```python
from build123d import *

# Parameters (mm, degrees)
F0_R     = 1.7272
F0_R_2   = 3.96875
F0_R_3   = 11.1125
F0_R_4   = 2.15265
F1_DEPTH = 3.175
F3_DEPTH = 3.175
F4_COUNT = 6
F4_ANGLE = 300


with BuildPart() as f1:
    # F0 (on Top) → F1 (new body)
    with BuildSketch(Plane.XY):
        with BuildLine():
            Line((-303.6125627, 32.54375), (-346.1094200534, 21.5120031198))
            ThreePointArc((-346.1094200534, 21.5120031198), (-362.7501254, 0), (-346.1094200534, -21.5120031198))
            Line((-346.1094200534, -21.5120031198), (-303.6125627, -32.54375))
            Line((-303.6125627, -32.54375), (-297.2625627, -32.54375))
            Line((-297.2625627, -32.54375), (-297.2625627, -29.36875))
            Line((-297.2625627, -29.36875), (-43.2625627, -29.36875))
            Line((-43.2625627, -29.36875), (-43.2625627, -32.54375))
            Line((-43.2625627, -32.54375), (-36.9125627, -32.54375))
            Line((-36.9125627, -32.54375), (5.5842946534, -21.5120031198))
            ThreePointArc((5.5842946534, -21.5120031198), (22.225, 0), (5.5842946534, 21.5120031198))
            Line((5.5842946534, 21.5120031198), (-36.9125627, 32.54375))
            Line((-36.9125627, 32.54375), (-43.2625627, 32.54375))
            Line((-43.2625627, 32.54375), (-43.2625627, 29.36875))
            Line((-43.2625627, 29.36875), (-297.2625627, 29.36875))
            Line((-297.2625627, 29.36875), (-297.2625627, 32.54375))
            Line((-297.2625627, 32.54375), (-303.6125627, 32.54375))
        make_face()
        with Locations((-282.9750627, -24.60625)):
            Circle(F0_R, mode=Mode.SUBTRACT)
        with Locations((-352.3117115589, -11.7865861589)):
            Circle(F0_R, mode=Mode.SUBTRACT)
        with Locations((-328.7385392411, -11.7865861589)):
            Circle(F0_R_2, mode=Mode.SUBTRACT)
        with Locations((-57.5500627, -24.60625)):
            Circle(F0_R, mode=Mode.SUBTRACT)
        with Locations((-11.7865861589, -11.7865861589)):
            Circle(F0_R_2, mode=Mode.SUBTRACT)
        with Locations((11.7865861589, -11.7865861589)):
            Circle(F0_R, mode=Mode.SUBTRACT)
        with Locations((-340.5251254, 0)):
            Circle(F0_R_3, mode=Mode.SUBTRACT)
        with Locations((-289.7251254, 0)):
            Circle(F0_R_4, mode=Mode.SUBTRACT)
        with Locations((-352.3117115589, 11.7865861589)):
            Circle(F0_R_2, mode=Mode.SUBTRACT)
        with Locations((-328.7385392411, 11.7865861589)):
            Circle(F0_R, mode=Mode.SUBTRACT)
        with Locations((-282.9750627, 24.60625)):
            Circle(F0_R, mode=Mode.SUBTRACT)
        with Locations((-50.8, 0)):
            Circle(F0_R_4, mode=Mode.SUBTRACT)
        Circle(F0_R_3, mode=Mode.SUBTRACT)
        with Locations((-11.7865861589, 11.7865861589)):
            Circle(F0_R, mode=Mode.SUBTRACT)
        with Locations((11.7865861589, 11.7865861589)):
            Circle(F0_R_2, mode=Mode.SUBTRACT)
        with Locations((-57.5500627, 24.60625)):
            Circle(F0_R, mode=Mode.SUBTRACT)
    extrude(amount=F1_DEPTH)

    # F2 (on face) → F3 (cut, through all)
    with BuildSketch(Plane(origin=(0, 0, 0), x_dir=(1, 0, 0), z_dir=(0, 0, -1))):
        with BuildLine():
            ThreePointArc((-348.3828495059, -7.8577241059), (-350.1488326996, -5.55625), (-351.2589761446, -2.8761266387))
            Line((-351.2589761446, -2.8761266387), (-352.0256797693, -3.0815642558))
            ThreePointArc((-352.0256797693, -3.0815642558), (-350.8362403638, -5.953125), (-348.9441155135, -8.4189901135))
            Line((-348.9441155135, -8.4189901135), (-348.3828495059, -7.8577241059))
        make_face()
    f3 = extrude(amount=-F3_DEPTH, mode=Mode.SUBTRACT)

    # F4: F3 ×6 about axis
    f4_axis = Axis((-340.5251254, 0, 0), (0, 0, -1))
    for i in range(1, F4_COUNT):
        add(f3.rotate(f4_axis, i * F4_ANGLE / (F4_COUNT - 1)), mode=Mode.SUBTRACT)


solid = f1.part
```
Here's how the part is built. I have some questions about the finished solid (model axes, mm). Give positions to 0.01 mm unless a question says otherwise; leave off trailing zeros. Order: outer loops, then holes, each group sorted by start corner. A loop starts at its lowest first (then second) coordinate and runs counter-clockwise, first axis right, second up. Notation, with made-up numbers: M 45,-4.5 L 72,-4.5 A28 ccw 72,34.5 Z; hole C 65.5,-12 d10. An arc over 180 degrees is marked long. Use a Markdown table: item, result. Add a question column.
1. I need wall thicknesses on probe 1 along Y at (x, z) = (0.5, 0.8); probe 2 along X at (y, z) = (0.5, 2.95); probe 3 along X at (y, z) = (5, 1.5). Which ranges of each line are inside material? Lowest first, please. Write a range as from..to.
2. Suppose I cut it at A-A (x = 0). List the corners of the cut face in (y, z) for me (1 decimal).
3. Suppose I cut it at B-B (z = 1.7). Give the number of separate pieces and of enclosed holes in the cut face, and give its area (3 significant figures).
4. Suppose I cut it at C-C (x = -207.5). List the corners of the cut face in (y, z) for me (3 decimals), and give its area (3 significant figures).
5. If we mould it in two halves opening along Z, with no side actions, what happens to faces 1 (the cylindrical face through (10.6, 3.34, 1.57)), 2 (the flat face through (-173, 0, 3.175)), 3 (the flat face through (-173, 0, 0))? For each: +Z half, -Z half, draft (parallel to the pull), parting line (faces both ways), or undercut.
6. For pin 1 Ø5.5 at (x, y) = (-282.98, 24.61) entering from -Z; pin 2 Ø18 at (x, y) = (0, 0) entering from -Z, each with a flat end and sliding along its axis, tell me the tip position at first contact or that it passes through.
Results list:
| question | item | result |
|---|---|---|
| 1 | probe 1 | y = -22.83..-11.1, 11.1..22.83 |
| 1 | probe 2 | x = -362.74..-351.63, -329.42..-291.82, -287.63..-52.89, -48.71..-11.1, 11.1..22.22 |
| 1 | probe 3 | x = -362.18..-351.33, -329.72..-9.92, 9.92..21.66 |
| 2 | outline | M -23,0 L -11.1,0 L -11.1,3.2 L -23,3.2 Z; M 11.1,0 L 23,0 L 23,3.2 L 11.1,3.2 Z |
| 3 | separate pieces | 1 |
| 3 | enclosed holes | 16 |
| 3 | area | 20,300 mm² |
| 4 | outline | M -29.369,0 L 29.369,0 L 29.369,3.175 L -29.369,3.175 Z |
| 4 | area | 186 mm² |
| 5 | face 1 | draft |
| 5 | face 2 | +Z half |
| 5 | face 3 | -Z half |
| 6 | pin 1 | stops at z = 0 |
| 6 | pin 2 | passes through |
